Geometry check sheet. Reference: drawing and pictorial views, mm from the part's lowest x, y, z. A direction names the side the tool comes from. Round coordinates to 2 decimals unless told otherwise and drop trailing zeros. Order: outer loops, then holes, each group sorted by start corner. A loop starts at its lowest first (then second) coordinate and runs counter-clockwise, first axis right, second up. Notation, with made-up numbers: (26.25, 3.5) -> (82.25, 3.5) arc R6 cw to (82.25, 11.5) -> close; hole circle Ø7 at (8, 5.25). An arc over 180 degrees is marked (long way). Return JSON: item names as keys, results as strings. Group by question number.
1) Section check B-B on x = 25. Enter the section's corners in (y, z).
2) Section check D-D on y = 28. Enter the section's corners in (x, z).
3) Tool access check on the marked faces 1 and 2. Record the directions out of +Z, -Z, +X, -X, +Y, -Y that give a thin tool (end or side, any length) a straight path to the whole face; none if there is none.
4) Depth check by flat-ended pin: pin 1 (1 mm diameter, centred on x = 23.5, z = 6, fed in from -Y); pin 2 (12 mm diameter, centred on x = 29.5, y = 14, fed in from +Z); pin 3 (10 mm diameter, centred on y = 32.5, z = 13.5, fed in from +X). Enter the tip coordinate at first touch or a pass-through.
5) Section check A-A on z = 20.5. Enter the section's corners in (x, y).
6) Section check C-C on x = 17. Enter the section's corners in (y, z).
7) Scan lines: L1, parallel to Z at x = 28, y = 20.5; L2, parallel to Y at x = 3.5, z = 4. Record each from-to range of solid material in increasing order.
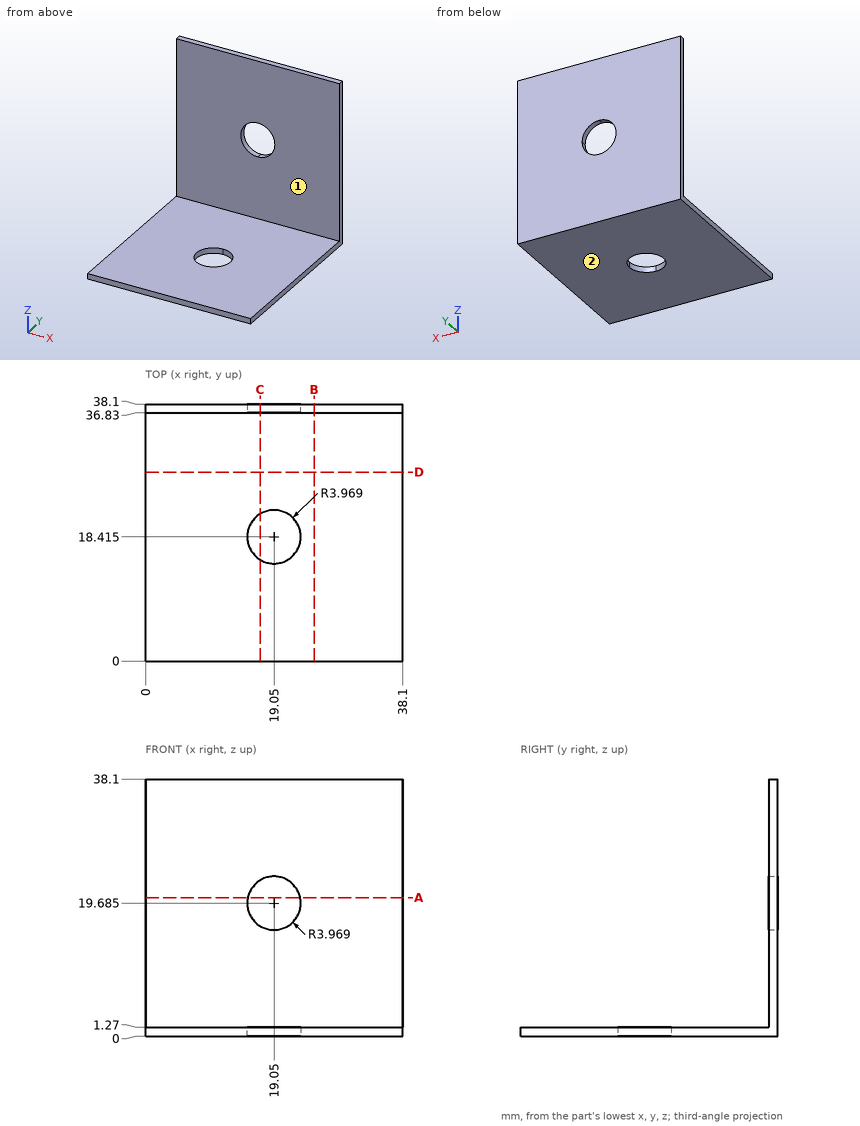
Check result:
{
 "1": {"outline": "(0, 0) -> (38.1, 0) -> (38.1, 38.1) -> (36.83, 38.1) -> (36.83, 1.27) -> (0, 1.27) -> close"},
 "2": {"outline": "(0, 0) -> (38.1, 0) -> (38.1, 1.27) -> (0, 1.27) -> close"},
 "3": {"face 1": "+Z, +X, -X, -Y", "face 2": "-Z, +X, -X, +Y, -Y"},
 "4": {"pin 1": "y = 36.83", "pin 2": "z = 1.27", "pin 3": "x = 38.1"},
 "5": {"outline": "(0, 36.83) -> (15.17, 36.83) -> (15.17, 38.1) -> (0, 38.1) -> close; (22.93, 36.83) -> (38.1, 36.83) -> (38.1, 38.1) -> (22.93, 38.1) -> close"},
 "6": {"outline": "(0, 0) -> (15.02, 0) -> (15.02, 1.27) -> (0, 1.27) -> close; (21.81, 0) -> (38.1, 0) -> (38.1, 16.29) -> (36.83, 16.29) -> (36.83, 1.27) -> (21.81, 1.27) -> close; (36.83, 23.08) -> (38.1, 23.08) -> (38.1, 38.1) -> (36.83, 38.1) -> close"},
 "7": {"L1": "0 to 1.27", "L2": "36.83 to 38.1"}
}
